Autodesk Inventor part; units mm, degrees
ref_plane "YZ Plane" through (0, 0, 0) normal (1, 0, 0) x (0, 1, 0)
ref_plane "XZ Plane" through (0, 0, 0) normal (0, 1, 0) x (-1, 0, 0)
ref_plane "XY Plane" through (0, 0, 0) normal (0, 0, 1) x (1, 0, 0)
sketch "Sketch1" plane through (0, 0, 0) normal (0, 0, 1) x (1, 0, 0)
  arc A0 (2.287945, 4.093737) -> (-3.198455, 4.093737) centre (-0.455255, 4.093737) ccw
  arc A1 (-3.198455, -3.119863) -> (2.287945, -3.119863) centre (-0.455255, -3.119863) ccw
  line L0 (-3.198455, 4.093737) -> (-3.198455, -3.119863)
  line L1 (2.287945, 4.093737) -> (2.287945, -3.119863)
  arc A2 (1.525945, 4.093737) -> (-2.436455, 4.093737) centre (-0.455255, 4.093737) ccw
  line L2 (1.525945, 4.093737) -> (1.525945, -3.119863)
  arc A3 (-2.436455, -3.119863) -> (1.525945, -3.119863) centre (-0.455255, -3.119863) ccw
  line L3 (-2.436455, -3.119863) -> (-2.436455, 4.093737)
  point P0 (0, 0)
  dimension "d0" = 5.4864
  dimension "d1" = 5.4864
  dimension "d3" = 12.7
  dimension "d4" = 0.762
extrude "Extrusion1" add sketch "Sketch1" along normal mid plane 2.032
sketch "Sketch2" plane through (0, 0, 1.016) normal (0, 0, 1) x (1, 0, 0)
  line L0 (1.525945, -3.119863) -> (1.525945, 4.093737)
  arc A0 (1.525945, 4.093737) -> (-2.436455, 4.093737) centre (-0.455255, 4.093737) ccw
  line L1 (-2.436455, 4.093737) -> (-2.436455, -3.119863)
  arc A1 (-2.436455, -3.119863) -> (1.525945, -3.119863) centre (-0.455255, -3.119863) ccw
  line L2 (2.287945, 4.093737) -> (2.287945, -3.119863)
  arc A2 (-3.198455, -3.119863) -> (2.287945, -3.119863) centre (-0.455255, -3.119863) ccw
  line L3 (-3.198455, -3.119863) -> (-3.198455, 4.093737)
  arc A3 (2.287945, 4.093737) -> (-3.198455, 4.093737) centre (-0.455255, 4.093737) ccw
  arc A4 (3.697645, 4.093737) -> (-4.608155, 4.093737) centre (-0.455255, 4.093737) ccw
  line L4 (3.697645, 4.093737) -> (3.697645, -3.119863)
  arc A5 (-4.608155, -3.119863) -> (3.697645, -3.119863) centre (-0.455255, -3.119863) ccw
  line L5 (-4.608155, -3.119863) -> (-4.608155, 4.093737)
  point P0 (0, 0)
  dimension "d7" = 8.3058
sketch "Sketch2 outline for Extrusion2" plane through (0, 0, 1.016) normal (0, 0, 1) x (1, 0, 0)
  arc A0 (-4.608155, 4.093737) -> (3.697645, 4.093737) centre (-0.455255, 4.093737) cw
  line L0 (-4.608155, -3.119863) -> (-4.608155, 4.093737)
  line L1 (3.697645, 4.093737) -> (3.697645, -3.119863)
  arc A1 (3.697645, -3.119863) -> (-4.608155, -3.119863) centre (-0.455255, -3.119863) cw
  arc A2 (-2.436455, -3.119863) -> (1.525945, -3.119863) centre (-0.455255, -3.119863) ccw
  line L2 (1.525945, -3.119863) -> (1.525945, 4.093737)
  arc A3 (1.525945, 4.093737) -> (-2.436455, 4.093737) centre (-0.455255, 4.093737) ccw
  line L3 (-2.436455, 4.093737) -> (-2.436455, -3.119863)
extrude "Extrusion2" add sketch "Sketch2 outline for Extrusion2" along normal blind 1.27 draft -15
mirror "Mirror1" about plane through (0, 0, 0) normal (0, 0, 1) of "Extrusion2"
properties part number "Nibblets"
Part model, mm, in its own coordinate system. A direction names the side the tool comes from. Give positions to 0.01 mm unless a question says otherwise; leave off trailing zeros. Write each loop counter-clockwise with the first axis right and the second up, starting at its lowest first coordinate (ties: lowest second). Pieces come first, ordered by that corner, then holes.
1) Cut at A-A on z = -0.55. Write the cut outline in (x, y), then the cut area to 3 significant figures.
Resolved:
outline: (-3.2, -3.12) arc R2.74 ccw to (2.29, -3.12) - (2.29, 4.09) arc R2.74 ccw to (-3.2, 4.09) - close; hole (-2.44, -3.12) arc R1.98 ccw to (1.53, -3.12) - (1.53, 4.09) arc R1.98 ccw to (-2.44, 4.09) - close
area: 22.3 mm2
2) Cut at B-B on y = 3. Write the cut outline in (x, z), then the cut area to 3 significant figures.
Resolved:
outline: (-4.61, -1.02) - (-4.27, -2.29) - (-2.78, -2.29) - (-2.44, -1.02) - (-2.44, 1.02) - (-2.78, 2.29) - (-4.27, 2.29) - (-4.61, 1.02) - (-3.2, 1.02) - (-3.2, -1.02) - close; (1.53, -1.02) - (1.87, -2.29) - (3.36, -2.29) - (3.7, -1.02) - (2.29, -1.02) - (2.29, 1.02) - (3.7, 1.02) - (3.36, 2.29) - (1.87, 2.29) - (1.53, 1.02) - close
area: 12.4 mm2
3) Which spindle directions (+Z, -Z, +X, -X, +Y, -Y) get a long thin tool onto all of the face, cutting with end or side? Do faces 1 (the face through (-0.41, 6.21, 1.52)), 2 (the face through (1.694, 0.537, -1.642)), 3 (the face through (-0.4, -5.1, 0)). Say none if no direction does.
Resolved:
face 1: +Z
face 2: -Z
face 3: +Z, -Z
4) Pin check, flat tips, straight feed: pin 1 (1.6 mm diameter, centred on y = 1, z = -0.5, fed in from -X); pin 2 (2 mm diameter, centred on x = -3.5, z = 1, fed in from -Y); pin 3 (0.6 mm diameter, centred on y = 0, z = 0, fed in from -X). Stop position of each tip, or through.
Resolved:
pin 1: stops at x = -4.61
pin 2: stops at y = -6.73
pin 3: stops at x = -3.2
5) Two-plate mould, pull along Z, no slides. Class faces 4 (the face through (1.694, 0.436, 1.642)), 5 (the face through (2.288, 1, 0)), 6 (the face through (-0.395, -5.862, -0.014)), 7 (the face through (-2.604, 0.436, -1.642)): released by +Z, released by -Z, zero draft, split by the parting line, or undercut.
Resolved:
face 4: released by +Z
face 5: undercut
face 6: undercut
face 7: released by -Z
6) Probe L1, parallel to X at y = 3, z = -0.6; L2, parallel to Z at x = -4, y = 4; L3, parallel to X at y = -0.25, z = -1.65. List the from-to ranges inside material, lowest first.
Resolved:
L1: x = -3.2 to -2.44, 1.53 to 2.29
L2: z = -2.29 to -1.02, 1.02 to 2.29
L3: x = -4.44 to -2.61, 1.7 to 3.53
